The listing builds one solid part. Answer for the finished solid, in the listing's coordinates (mm). Face numbers are marked on the shaded views. A direction names the side the tool comes from. Coordinates: 2 decimals unless noted, no trailing zeros. Loops run counter-clockwise (first coordinate to the right, second up) from the corner with the lowest first, then second, coordinate; pieces in that order, holes last. Notation, with made-up numbers: M 64,82 L 99,82 A20 cw 99,113 Z; hole C 77,37 d1. An arc over 180 degrees is marked long. Return JSON: item names as keys, results as strings. Group by question number.
1. Section B-B (x = 0) is taken. Write down the section's boundary in (y, z) (3 decimals).
2. Section A-A (z = 0) is taken. Write down the section's boundary in (x, y) (3 decimals), then the cut area to 3 significant figures.
3. Given P1, Ø3, axis at x = -19.5, z = -5.5, coming from the +Y side; P2, Ø5, axis at y = 6.5, z = 13, coming from the +X side; P3, Ø2, axis at x = -5.5, y = 2, coming from the +Z side, each flat-ended and moving along its own axis, determine where each tip first touches the part or whether it passes through.
4. Straight lines are drawn through the part: L1, parallel to Y at x = 15, z = 7.5; L2, parallel to X at y = 0.75, z = 1.5; L3, parallel to Z at x = 4, y = 7.25. For each, find the intervals that lie inside material, in ascending order. Write a range as from..to.
5. Which of the six approach directions +Z, -Z, +X, -X, +Y, -Y give full straight-line access (tool end or side, diameter ignored) to the marked faces 1 and 2?
6. Section C-C (y = 8) is taken. Write down the section's boundary in (x, z).
7. Section D-D (y = 4.25) is taken. Write down the section's boundary in (x, z), then the cut area to 3 significant figures.
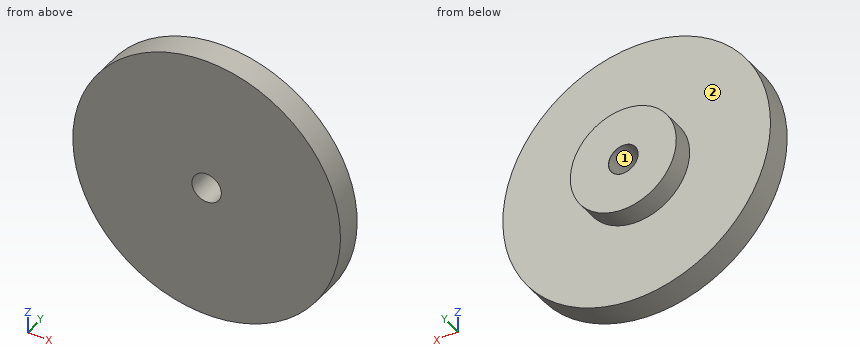
```python
from build123d import *

# Parameters (mm, degrees)
SKETCH1_R                      = 25
BOSS_EXTRUDE1_DEPTH            = 5
SKETCH2_R                      = 9.9
BOSS_EXTRUDE2_DEPTH            = 4
M5_CLEARANCE_HOLE1_D           = 5.5
M5_CLEARANCE_HOLE1_CSINK_D     = 5.55
M5_CLEARANCE_HOLE1_CSINK_ANGLE = 90


with BuildPart() as part:
    # Sketch1 → Boss-Extrude1 (new body)
    with BuildSketch(Plane(origin=(0, 0, 0), x_dir=(1, 0, 0), z_dir=(0, 1, 0))):
        with Locations(Location((0, 0, 0), (0, 0, 270))):
            Circle(SKETCH1_R)
    extrude(amount=BOSS_EXTRUDE1_DEPTH)

    # Sketch2 → Boss-Extrude2 (add)
    with BuildSketch(Plane(origin=(0, 5, 0), x_dir=(1, 0, 0), z_dir=(0, 1, 0))):
        with Locations(Location((0, 0, 0), (0, 0, 270))):
            Circle(SKETCH2_R)
    extrude(amount=BOSS_EXTRUDE2_DEPTH)

    # M5 Clearance Hole1 (through all)
    with Locations(Plane(origin=(0, 9, 0), x_dir=(1, 0, 0), z_dir=(0, 1, 0))):
        with Locations((0, 0)):
            CounterSinkHole(M5_CLEARANCE_HOLE1_D / 2, M5_CLEARANCE_HOLE1_CSINK_D / 2, counter_sink_angle=M5_CLEARANCE_HOLE1_CSINK_ANGLE)


solid = part.part
```
Worked out:
{
 "1": {"outline": "M 0,-25 L 5,-25 L 5,-9.9 L 9,-9.9 L 9,-2.775 L 8.975,-2.75 L 0,-2.75 Z; M 0,2.75 L 8.975,2.75 L 9,2.775 L 9,9.9 L 5,9.9 L 5,25 L 0,25 Z"},
 "2": {"outline": "M -25,0 L -2.75,0 L -2.75,8.975 L -2.775,9 L -9.9,9 L -9.9,5 L -25,5 Z; M 2.75,0 L 25,0 L 25,5 L 9.9,5 L 9.9,9 L 2.775,9 L 2.75,8.975 Z", "area": "280 mm^2"},
 "3": {"P1": "y = 5", "P2": "x = 22.45", "P3": "z = 24.59"},
 "4": {"L1": "0..5", "L2": "-24.95..-2.3, 2.3..24.95", "L3": "-9.06..9.06"},
 "5": {"face 1": "+Y, -Y", "face 2": "+Y"},
 "6": {"outline": "C 0,0 d19.8; hole C 0,0 d5.5"},
 "7": {"outline": "C 0,0 d50; hole C 0,0 d5.5", "area": "1,940 mm^2"}
}
